```python
from build123d import *

# Parameters (mm, degrees)
F0_W     = 31.75
F0_H     = 31.75
F1_DEPTH = 2.032
F2_W     = 31.75
F2_H     = 31.75
F3_DEPTH = 2.032
F4_R     = 0.508
F5_R     = 1.27
F6_R     = 1.5875
F6_R_2   = 3.96875
F7_DEPTH = 25.4


with BuildPart() as f1:
    # F0 (on Top) → F1 (new body)
    with BuildSketch(Plane.XY):
        with Locations((-14.342583, -18.160402)):
            Rectangle(F0_W, F0_H)
    extrude(amount=F1_DEPTH)

    # F2 (on face) → F3 (join)
    with BuildSketch(Plane.XZ.offset(34.035402)):
        with Locations((-14.342583, 15.875)):
            Rectangle(F2_W, F2_H)
    extrude(amount=-F3_DEPTH)

    # F4
    f4_edges = [f1.edges().sort_by_distance(p)[0] for p in [
        (-14.342583, -32.003402, 2.032),
    ]]
    fillet(f4_edges, radius=F4_R)

    # F5
    f5_edges = [f1.edges().sort_by_distance(p)[0] for p in [
        (-14.342583, -34.035402, 0),
    ]]
    fillet(f5_edges, radius=F5_R)

    # F6 (on face) → F7 (cut)
    with BuildSketch(Plane.XY.offset(2.032)):
        with Locations((-14.342583, -9.079902)):
            Circle(F6_R)
        with Locations((-20.045045, -11.441939)):
            Circle(F6_R)
        with Locations((-22.407083, -17.144402)):
            Circle(F6_R)
        with Locations((-20.045045, -22.846864)):
            Circle(F6_R)
        with Locations((-14.342583, -25.208902)):
            Circle(F6_R)
        with Locations((-8.64012, -22.846864)):
            Circle(F6_R)
        with Locations((-6.278083, -17.144402)):
            Circle(F6_R)
        with Locations((-8.64012, -11.441939)):
            Circle(F6_R)
        with Locations((-14.342583, -17.144402)):
            Circle(F6_R_2)
    extrude(amount=-F7_DEPTH, mode=Mode.SUBTRACT)


solid = f1.part
```
For this review, take the finished solid that the model builds, in its own axes (mm). A direction names the side the tool comes from. Coordinates: 2 decimals unless noted, no trailing zeros. Write each loop counter-clockwise with the first axis right and the second up, starting at its lowest first coordinate (ties: lowest second). Pieces come first, ordered by that corner, then holes.
(1) Add section C-C on x = -23. Give the boundary of the cut face in (y, z), then the cut area to 3 significant figures.
(2) Tool access review of faces 1 (the face through (-18, -13, 2.032)), 2 (the face through (-8.847, -21.273, 1.03)): name each direction out of +Z, -Z, +X, -X, +Y, -Y from which nothing blocks a thin tool from reaching the whole face with its end or side.
(3) Add section D-D on y = -4.5. Give the boundary of the cut face in (x, z), then the cut area to 3 significant figures.
(4) Add section B-B on x = 0. Give the boundary of the cut face in (y, z).
(5) Wall thickness on probe 1 along Y at (x, z) = (-20, 7); probe 2 along Z at (x, y) = (-11, -20); probe 3 along Y at (x, z) = (-21.5, 1): over which ranges is each line inside the solid? List them lowest first.
(6) For pin 1 Ø14.5 at (x, z) = (-11, 10) entering from +Y; pin 2 Ø9 at (x, y) = (-18, -14.5) entering from +Z, all flat-tipped, find the tip position at first contact; note any pin that passes through.
(7) Add section A-A on y = -19.5. Give the boundary of the cut face in (x, z).
Answer sheet:
1. outline: (-34.04, 1.27) arc R1.27 ccw to (-32.77, 0) - (-18.62, 0) - (-18.62, 2.03) - (-31.5, 2.03) arc R0.51 cw to (-32, 2.54) - (-32, 31.75) - (-34.04, 31.75) - close; (-15.67, 0) - (-2.29, 0) - (-2.29, 2.03) - (-15.67, 2.03) - close
1. area: 119 mm2
2. face 1: +Z, +X, -X, +Y
2. face 2: +Z, -Z
3. outline: (-30.22, 0) - (1.53, 0) - (1.53, 2.03) - (-30.22, 2.03) - close
3. area: 64.5 mm2
4. outline: (-34.04, 1.27) arc R1.27 ccw to (-32.77, 0) - (-2.29, 0) - (-2.29, 2.03) - (-31.5, 2.03) arc R0.51 cw to (-32, 2.54) - (-32, 31.75) - (-34.04, 31.75) - close
5. probe 1: y = -34.04 to -32
5. probe 2: z = 0 to 2.03
5. probe 3: y = -34.01 to -23.48, -22.21 to -18.45, -15.84 to -12.08, -10.81 to -2.29
6. pin 1: stops at y = -32
6. pin 2: stops at z = 2.03
7. outline: (-30.22, 0) - (-17.54, 0) - (-17.54, 2.03) - (-30.22, 2.03) - close; (-11.15, 0) - (1.53, 0) - (1.53, 2.03) - (-11.15, 2.03) - close
